For this review, take the finished solid that the model builds, in its own axes (mm). Coordinates: 2 decimals unless noted, no trailing zeros. Write each loop counter-clockwise with the first axis right and the second up, starting at its lowest first coordinate (ties: lowest second). Pieces come first, ordered by that corner, then holes. Notation, with made-up numbers: M 51.25,74 L 83.25,74 A15 cw 83.25,85 Z; hole C -20,45 d1. An arc over 180 degrees is marked long. Return JSON: item names as keys, results as strings.
```python
from build123d import *

# Parameters (mm, degrees)
F0_W     = 500
F0_H     = 250
F1_DEPTH = 6.35
F2_W     = 50
F2_H     = 3.175
F2_W_2   = 3.175
F2_H_2   = 25
F3_DEPTH = 6.351


# Not quite as in the source:
# - a length typed as a fraction of an inch, garbled in the dataset ("3 / 203.2 mm" for 3/8 in), is restored


with BuildPart() as f1:
    # F0 (on Top) → F1 (new body)
    with BuildSketch(Plane.XY):
        Rectangle(F0_W, F0_H)
    extrude(amount=F1_DEPTH)

    # F2 (on face) → F3 (cut, through all)
    with BuildSketch(Plane.XY.offset(6.35)):
        with Locations((-200, 123.4125)):
            Rectangle(F2_W, F2_H)
        with Locations((-200, -123.4125)):
            Rectangle(F2_W, F2_H)
        with Locations((-100, 123.4125)):
            Rectangle(F2_W, F2_H)
        with Locations((-100, -123.4125)):
            Rectangle(F2_W, F2_H)
        with Locations((0, 123.4125)):
            Rectangle(F2_W, F2_H)
        with Locations((0, -123.4125)):
            Rectangle(F2_W, F2_H)
        with Locations((100, 123.4125)):
            Rectangle(F2_W, F2_H)
        with Locations((100, -123.4125)):
            Rectangle(F2_W, F2_H)
        with Locations((200, 123.4125)):
            Rectangle(F2_W, F2_H)
        with Locations((200, -123.4125)):
            Rectangle(F2_W, F2_H)
        with Locations((248.4125, 87.5)):
            Rectangle(F2_W_2, F2_H_2)
        with Locations((248.4125, 29.1666666667)):
            Rectangle(F2_W_2, F2_H_2)
        with Locations((248.4125, -29.1666666667)):
            Rectangle(F2_W_2, F2_H_2)
        with Locations((248.4125, -87.5)):
            Rectangle(F2_W_2, F2_H_2)
        with Locations((-248.4125, -87.5)):
            Rectangle(F2_W_2, F2_H_2)
        with Locations((-248.4125, 29.1666666667)):
            Rectangle(F2_W_2, F2_H_2)
        with Locations((-248.4125, -29.1666666667)):
            Rectangle(F2_W_2, F2_H_2)
        with Locations((-248.4125, 87.5)):
            Rectangle(F2_W_2, F2_H_2)
    extrude(amount=-F3_DEPTH, mode=Mode.SUBTRACT)


solid = f1.part
```
1. We need section A-A (x = 200.5). State the section outline as (y, z) points (3 decimals), plus the area to 3 significant figures.
Checks:
{"outline": "M -121.825,0 L 121.825,0 L 121.825,6.35 L -121.825,6.35 Z", "area": "1,550 mm2"}
2. Clearance check with flat-ended pins moving along their axes: pin 1 Ø3 at (y, z) = (-31, 1.5) entering from -X (3 decimals); pin 2 Ø1 at (x, z) = (-123, 4) entering from +Y (3 decimals); pin 3 Ø3 at (x, y) = (94, -25.5) entering from -Z. State where each tip first meets the part, or that it passes through.
Checks:
{"pin 1": "x = -246.825", "pin 2": "y = 121.825", "pin 3": "z = 0"}
3. Wall thickness on L1, parallel to Y at x = 17.5, z = 2.75 (3 decimals); L2, parallel to X at y = -40, z = 5 (3 decimals): over which ranges is each line inside the solid? List them lowest first. Write a range as from..to.
Checks:
{"L1": "-121.825..121.825", "L2": "-246.825..246.825"}
